Source: CAD feature listing. Evaluate the final solid. Frame: model axes, mm. A direction names the side the tool comes from. Round coordinates to 2 decimals unless told otherwise and drop trailing zeros. Order: outer loops, then holes, each group sorted by start corner. A loop starts at its lowest first (then second) coordinate and runs counter-clockwise, first axis right, second up. Notation, with made-up numbers: (9, 80.5) - (17, 80.5) arc R14 ccw to (17, 90.5) - close; hole circle Ø5 at (71.25, 12.5). An arc over 180 degrees is marked (long way). Put each result on its own line as item: value. Start each with the question number.
1) Section C-C on y = 81.5. Output: boundary loops of the cut face in (x, z), then the cut area to 3 significant figures.
2) Section D-D on y = 226. Output: boundary loops of the cut face in (x, z).
3) Section B-B on x = 0. Output: boundary loops of the cut face in (y, z).
4) Section A-A on z = 0. Output: boundary loops of the cut face in (x, y), then the cut area to 3 significant figures.
5) Access query for faces 1 (the face through (-208, 625, 430)), 2 (the face through (14, 0, -14)), 3 (the face through (-50, 63, -3)). Directions: +Z, -Z, +X, -X, +Y, -Y. A direction counts if a zero-diameter tool reaches every point of the face in a straight line with its end or side. Return the directions, or none.
6) Line query: probe 1 along X at (y, z) = (346, 0); probe 2 along Y at (x, z) = (-705.5, 236); probe 3 along X at (y, z) = (252.5, 57). Output: solid intervals per line, ascending. Write a range as [from, to].
7) Mould query, pull axis X, two halves, no side actions, for faces 4 (the face through (172, 1000, 78)), 5 (the face through (0, 125, -3)), 6 (the face through (48.088, 63, 3)), 7 (the face through (371.81, 860.58, -48.82)). Classes: +X half, -X half, draft (parallel to the pull), parting line (faces both ways), or undercut.
8) Contact query for flat-ended pins moving along their axis: P1, Ø12, axis at x = 771, y = 482.5, coming from the -Z side; P2, Ø2, axis at y = 768.5, z = -295, coming from the +X side; P3, Ø2, axis at y = 287, z = -640, coming from the -X side. Output: stop coordinate, or through.
```python
from build123d import *

# Parameters (mm, degrees)
SKETCH1_R           = 1000
BOSS_EXTRUDE1_DEPTH = 625
SKETCH2_R           = 375
BOSS_EXTRUDE2_DEPTH = 375
FILLET1_R           = 100
SKETCH3_R           = 187.5
CUT_EXTRUDE1_DEPTH  = 875
CUT_EXTRUDE2_START  = -125
CUT_EXTRUDE2_DEPTH  = 125


with BuildPart() as part:
    # Sketch1 → Boss-Extrude1 (new body)
    with BuildSketch(Plane(origin=(0, 0, 0), x_dir=(1, 0, 0), z_dir=(0, 1, 0))):
        with Locations(Location((0, 0, 0), (0, 0, 270))):
            Circle(SKETCH1_R)
    extrude(amount=BOSS_EXTRUDE1_DEPTH)

    # Sketch2 → Boss-Extrude2 (add)
    with BuildSketch(Plane(origin=(0, 625, 0), x_dir=(1, 0, 0), z_dir=(0, 1, 0))):
        with Locations(Location((0, 0, 0), (0, 0, 270))):
            Circle(SKETCH2_R)
    extrude(amount=BOSS_EXTRUDE2_DEPTH)

    # Fillet1
    fillet1_edges = [part.edges().sort_by_distance(p)[0] for p in [
        (0, 625, -375),
    ]]
    fillet(fillet1_edges, radius=FILLET1_R)

    # Sketch3 → Cut-Extrude1 (cut)
    with BuildSketch(Plane(origin=(0, 1000, 0), x_dir=(1, 0, 0), z_dir=(0, 1, 0))):
        with Locations(Location((0, 0, 0), (0, 0, 270))):
            Circle(SKETCH3_R)
    extrude(amount=-CUT_EXTRUDE1_DEPTH, mode=Mode.SUBTRACT)

    # Sketch4 → Cut-Extrude2 (cut)
    with BuildSketch(Plane(origin=(0, 0, 0), x_dir=(-1, 0, 0), z_dir=(0, -1, 0)).offset(CUT_EXTRUDE2_START)):
        with BuildLine():
            Line((50, 180.710403685), (50, -180.710403685))
            ThreePointArc((50, -180.710403685), (187.5, 0), (50, 180.710403685))
        make_face()
        with BuildLine():
            ThreePointArc((-48.087593772, 181.228676884), (-187.5, 0), (-48.087593772, -181.228676884))
            Line((-48.087593772, -181.228676884), (-48.087593772, 181.228676884))
        make_face()
    extrude(amount=CUT_EXTRUDE2_DEPTH, mode=Mode.SUBTRACT)


solid = part.part
```
Answer sheet:
1. outline: circle Ø2000 at (0, 0); hole (-50, -180.71) - (-50, 180.71) arc R187.5 ccw to start; hole (48.09, -181.23) arc R187.5 ccw to (48.09, 181.23) - close
1. area: 3,070,000 mm^2
2. outline: circle Ø2000 at (0, 0); hole circle Ø375 at (0, 0)
3. outline: (0, -1000) - (625, -1000) - (625, -475) arc R100 cw to (725, -375) - (1000, -375) - (1000, -187.5) - (125, -187.5) - (125, 187.5) - (1000, 187.5) - (1000, 375) - (725, 375) arc R100 cw to (625, 475) - (625, 1000) - (0, 1000) - close
4. outline: (-1000, 0) - (-187.5, 0) - (-187.5, 1000) - (-375, 1000) - (-375, 725) arc R100 cw to (-475, 625) - (-1000, 625) - close; (-50, 0) - (48.09, 0) - (48.09, 125) - (-50, 125) - close; (187.5, 0) - (1000, 0) - (1000, 625) - (475, 625) arc R100 cw to (375, 725) - (375, 1000) - (187.5, 1000) - close
4. area: 1,170,000 mm^2
5. face 1: +Y
5. face 2: +Z, -Z, +X, -X, -Y
5. face 3: +Y, -Y
6. probe 1: [-1000, -187.5], [187.5, 1000]
6. probe 2: [0, 625]
6. probe 3: [-998.37, -178.63], [178.63, 998.37]
7. face 4: draft
7. face 5: undercut
7. face 6: undercut
7. face 7: parting line
8. P1: z = -644.03
8. P2: x = 232.79
8. P3: x = -769.21
